Autodesk Inventor part; units mm, degrees
ref_plane "YZ Plane" through (0, 0, 0) normal (1, 0, 0) x (0, 1, 0)
ref_plane "XZ Plane" through (0, 0, 0) normal (0, 1, 0) x (-1, 0, 0)
ref_plane "XY Plane" through (0, 0, 0) normal (0, 0, 1) x (1, 0, 0)
sketch "Esboço1" plane through (0, 0, 0) normal (0, 0, 1) x (1, 0, 0)
  circle A0 centre (0, 0) radius 25
  dimension "d0" = 50
extrude "Extrusão1" add sketch "Esboço1" along normal blind 240
sketch "Esboço2" plane through (0, 0, 240) normal (0, 0, 1) x (1, 0, 0)
  circle A0 centre (0, 0) radius 30
  dimension "d3" = 60
extrude "Extrusão2" add sketch "Esboço2" along normal blind 50
chamfer "Chanfro1" distance 10 angle 45 1 edges at (-30, 0, 290)
thread "Rosca1"
sketch "Esboço3" plane through (0, 0, 0) normal (1, 0, 0) x (0, 1, 0)
  line L0 (30, 280) -> (-30, 280) construction
  line L1 (30, 240) -> (-30, 240) construction
  line L2 (30, 280) -> (-30, 240) construction
  line L3 (30, 240) -> (-30, 280) construction
  circle A0 centre (0, 260) radius 10
  point P0 (0, 0)
  dimension "d11" = 20
extrude "Extrusão3" cut sketch "Esboço3" along normal through all both and the other way through all
sketch "Esboço4" plane through (0, 0, 0) normal (0, 0, -1) x (-1, 0, 0)
  circle A0 centre (0, 0) radius 10
  dimension "d14" = 20
extrude "Extrusão4" add sketch "Esboço4" along normal blind 15
properties part number "Prisioneiro"
Input: part model. Units: mm. Frame: model coordinates. A direction names the side the tool comes from. Give positions to 0.01 mm unless a question says otherwise; leave off trailing zeros. Loops run counter-clockwise (first coordinate to the right, second up) from the corner with the lowest first, then second, coordinate; pieces in that order, holes last. Notation, with made-up numbers: (-39, 10.25) -> (-16, 10.25) arc R20 cw to (-16, 14.25) -> close; hole circle Ø10 at (68, 53.25). An arc over 180 degrees is marked (long way). Answer as a JSON object with one key per item and string values. Group by question number.
Item 1: Pull-direction query (Y, two-part tool) for faces 3 (the flat face through (-7, 25, 240)), 4 (the cylindrical face through (2.17, 9.76, -7.4)), 5 (the cylindrical face through (0.42, -1.302, 269.915)); classes: released by +Y, released by -Y, zero draft, split by the parting line, or undercut.
Item 2: Cut plane B-B, the plane x = 0. Return the cut outline in (y, z), and give its area (3 significant figures).
Item 3: Reachability of faces 1 (the flat face through (0, -11, 0)), 2 (the flat face through (0, 0, -15)) from +Z, -Z, +X, -X, +Y, -Y: full face, straight path, thin tool, end or side. Return the list, or none.
Item 4: Cut plane A-A, the plane y = 0. Return the cut outline in (x, z).
Item 5: Cut plane C-C, the plane z = 234. Return the cut outline in (x, y), and give its area (3 significant figures).
Item 6: Line query: probe 1 along Z at (x, y) = (14.5, 0); probe 2 along Z at (x, y) = (7.5, 0); probe 3 along Y at (x, z) = (13, 264). Output: solid intervals per line, ascending.
Item 7: Pin query (flat end, axial travel): P1, Ø3, axis at y = -1.5, z = 30, coming from the -X side; P2, Ø8, axis at x = 20.5, z = 193, coming from the +Y side; P3, Ø4, axis at y = -5.5, z = 25, coming from the -X side. Return the tip coordinate at first contact, or that it passes through.
Checks:
{
 "1": {"face 3": "zero draft", "face 4": "split by the parting line", "face 5": "undercut"},
 "2": {"outline": "(-30, 240) -> (-25, 240) -> (-25, 0) -> (-10, 0) -> (-10, -15) -> (10, -15) -> (10, 0) -> (25, 0) -> (25, 240) -> (30, 240) -> (30, 280) -> (20, 290) -> (-20, 290) -> (-30, 280) -> close; hole circle Ø20 at (0, 260)", "area": "14,900 mm²"},
 "3": {"face 1": "-Z", "face 2": "-Z, +X, -X, +Y, -Y"},
 "4": {"outline": "(-30, 240) -> (-25, 240) -> (-25, 0) -> (-10, 0) -> (-10, -15) -> (10, -15) -> (10, 0) -> (25, 0) -> (25, 240) -> (30, 240) -> (30, 250) -> (-30, 250) -> close; (-30, 270) -> (30, 270) -> (30, 280) -> (20, 290) -> (-20, 290) -> (-30, 280) -> close"},
 "5": {"outline": "circle Ø50 at (0, 0)", "area": "1,960 mm²"},
 "6": {"probe 1": "z = 0 to 250, 270 to 290", "probe 2": "z = -15 to 250, 270 to 290", "probe 3": "y = -27.04 to -9.17, 9.17 to 27.04"},
 "7": {"P1": "stops at x = -25", "P2": "stops at y = 18.78", "P3": "stops at x = -24.75"}
}
